```python
from build123d import *

# Parameters (mm, degrees)
SKETCH_1_W          = 100
SKETCH_1_H          = 35
EXTRUDE_1_DEPTH     = 1.6
CUT_EXTRUDE_1_DEPTH = 53.998207517
FILLET_1_R          = 3
SKETCH_3_W          = 12
SKETCH_3_H          = 6
EXTRUDE_2_DEPTH     = 6
SKETCH_4_R          = 3
EXTRUDE_3_DEPTH     = 10
SKETCH_5_W          = 4.5
SKETCH_5_H          = 6
SKETCH_5_W_2        = 5.403478788
SKETCH_5_H_2        = 11.06674021
EXTRUDE_4_DEPTH     = 2
SKETCH_6_W          = 7.585652914
SKETCH_6_H          = 2.805652448
SKETCH_6_W_2        = 13.612610022
EXTRUDE_5_DEPTH     = 2
SKETCH_7_W          = 9
SKETCH_7_H          = 4.5
EXTRUDE_6_DEPTH     = 6
CHAMFER_1_SIZE      = 2
SKETCH_9_R          = 0.65
CUT_EXTRUDE_2_DEPTH = 1
SWEEP_1_PROFILE_R   = 1.5
SKETCH_27_R         = 1.993301653
CUT_EXTRUDE_3_DEPTH = 1


with BuildPart() as part:
    # 草图1 → 凸台-拉伸1 (new body)
    with BuildSketch(Plane(origin=(0, 0, 0), x_dir=(1, 0, 0), z_dir=(0, 1, 0))):
        Rectangle(SKETCH_1_W, SKETCH_1_H)
    extrude(amount=EXTRUDE_1_DEPTH)

    # 草图2 → 切除-拉伸1 (cut, through all)
    with BuildSketch(Plane(origin=(0, 1.6, 0), x_dir=(1, 0, 0), z_dir=(0, 1, 0))):
        with BuildLine():
            Line((-49, 11), (-49, 15))
            ThreePointArc((-49, 15), (-47.5, 16.5), (-46, 15))
            Line((-46, 15), (-46, 11))
            ThreePointArc((-46, 11), (-47.5, 9.5), (-49, 11))
        make_face()
        with BuildLine():
            Line((49, 11), (49, 15))
            ThreePointArc((49, 15), (47.5, 16.5), (46, 15))
            Line((46, 15), (46, 11))
            ThreePointArc((46, 11), (47.5, 9.5), (49, 11))
        make_face()
        with BuildLine():
            Line((-49, -11), (-49, -15))
            ThreePointArc((-49, -15), (-47.5, -16.5), (-46, -15))
            Line((-46, -15), (-46, -11))
            ThreePointArc((-46, -11), (-47.5, -9.5), (-49, -11))
        make_face()
        with BuildLine():
            Line((49, -11), (49, -15))
            ThreePointArc((49, -15), (47.5, -16.5), (46, -15))
            Line((46, -15), (46, -11))
            ThreePointArc((46, -11), (47.5, -9.5), (49, -11))
        make_face()
    extrude(amount=-CUT_EXTRUDE_1_DEPTH, mode=Mode.SUBTRACT)

    # 圆角1
    fillet_1_edges = [part.edges().sort_by_distance(p)[0] for p in [
        (50, 0.8, 17.5),
        (-50, 0.8, 17.5),
        (-50, 0.8, -17.5),
        (50, 0.8, -17.5),
    ]]
    fillet(fillet_1_edges, radius=FILLET_1_R)

    # 草图3 → 凸台-拉伸2 (add)
    with BuildSketch(Plane(origin=(0, 1.6, 0), x_dir=(1, 0, 0), z_dir=(0, 1, 0))):
        with Locations((8, -14.5)):
            Rectangle(SKETCH_3_W, SKETCH_3_H)
    extrude(amount=EXTRUDE_2_DEPTH)

    # 草图4 → 凸台-拉伸3 (add)
    with BuildSketch(Plane(origin=(0, 7.6, 0), x_dir=(1, 0, 0), z_dir=(0, 1, 0))):
        with Locations(Location((8, -14.5, 0), (0, 0, 270))):
            Circle(SKETCH_4_R)
    extrude(amount=EXTRUDE_3_DEPTH)

    # 草图5 → 凸台-拉伸4 (add)
    with BuildSketch(Plane(origin=(0, 1.6, 0), x_dir=(1, 0, 0), z_dir=(0, 1, 0))):
        with Locations((-32.75, -2.5)):
            Rectangle(SKETCH_5_W, SKETCH_5_H)
        with Locations((-23.75, -2.5)):
            Rectangle(SKETCH_5_W, SKETCH_5_H)
        with Locations((-32.75, -12.5)):
            Rectangle(SKETCH_5_W, SKETCH_5_H)
        with Locations((-23.75, -12.5)):
            Rectangle(SKETCH_5_W, SKETCH_5_H)
        with Locations((-8.78065303, -7.299892016)):
            Rectangle(SKETCH_5_W_2, SKETCH_5_H_2)
        with Locations((23.75, -12.5)):
            Rectangle(SKETCH_5_W, SKETCH_5_H)
        with Locations((32.75, -12.5)):
            Rectangle(SKETCH_5_W, SKETCH_5_H)
        with Locations((32.75, -2.5)):
            Rectangle(SKETCH_5_W, SKETCH_5_H)
        with Locations((23.75, -2.5)):
            Rectangle(SKETCH_5_W, SKETCH_5_H)
    extrude(amount=EXTRUDE_4_DEPTH)

    # 草图6 → 凸台-拉伸5 (add)
    with BuildSketch(Plane(origin=(0, 1.6, 0), x_dir=(1, 0, 0), z_dir=(0, 1, 0))):
        with Locations((13.196957808, 8.988479137)):
            Rectangle(SKETCH_6_W, SKETCH_6_H)
        with Locations((-15.379131934, 8.988479137)):
            Rectangle(SKETCH_6_W_2, SKETCH_6_H)
    extrude(amount=EXTRUDE_5_DEPTH)

    # 草图7 → 凸台-拉伸6 (add)
    with BuildSketch(Plane(origin=(0, 1.6, 0), x_dir=(1, 0, 0), z_dir=(0, 1, 0))):
        with Locations((-28.25, 15.25)):
            Rectangle(SKETCH_7_W, SKETCH_7_H)
        with Locations((28.25, 15.25)):
            Rectangle(SKETCH_7_W, SKETCH_7_H)
        with Locations((-8.02152296, -15.25)):
            Rectangle(SKETCH_7_W, SKETCH_7_H)
    extrude(amount=EXTRUDE_6_DEPTH)

    # 倒角1
    chamfer_1_edges = [part.edges().sort_by_distance(p)[0] for p in [
        (-28.25, 7.6, -13),
        (28.25, 7.6, -13),
        (-8.02152296, 7.6, 13),
    ]]
    chamfer(chamfer_1_edges, length=CHAMFER_1_SIZE)

    # 草图9 → 切除-拉伸2 (cut)
    with BuildSketch(Plane(origin=(0, 7.6, 0), x_dir=(1, 0, 0), z_dir=(0, 1, 0))):
        with Locations(Location((-30.77012682, 16.126476079, 0), (0, 0, 270))):
            Circle(SKETCH_9_R)
        with Locations(Location((-25.898686841, 16.126476079, 0), (0, 0, 270))):
            Circle(SKETCH_9_R)
        with Locations(Location((25.614567714, 16.126476079, 0), (0, 0, 270))):
            Circle(SKETCH_9_R)
        with Locations(Location((30.638295355, 16.126476079, 0), (0, 0, 270))):
            Circle(SKETCH_9_R)
        with Locations(Location((-10.92906004, -16.309333864, 0), (0, 0, 270))):
            Circle(SKETCH_9_R)
        with Locations(Location((-5.225111254, -16.309333864, 0), (0, 0, 270))):
            Circle(SKETCH_9_R)
    extrude(amount=-CUT_EXTRUDE_2_DEPTH, mode=Mode.SUBTRACT)

    # 草图27 → 切除-拉伸3 (cut)
    with BuildSketch(Plane(origin=(0, 17.6, 0), x_dir=(1, 0, 0), z_dir=(0, 1, 0))):
        with Locations(Location((8, -14.5, 0), (0, 0, 270))):
            Circle(SKETCH_27_R)
    extrude(amount=-CUT_EXTRUDE_3_DEPTH, mode=Mode.SUBTRACT)


with BuildPart() as body_2:
    # 扫描1: sweep along a path in 草图10
    with BuildLine(Plane.XY.offset(14.5)) as sweep_1_path:
        Line((7.943335964, 14.862681463), (11, 26.862681463))
    # 扫描1 profile (on start of the path) → 扫描1 (sweep)
    with BuildSketch(Plane(origin=(7.943335964, 14.862681463, 14.5), x_dir=(0.9690562615876172, -0.24683995194828523, 0), z_dir=(0.24683995194828523, 0.9690562615876172, 0))):
        Circle(SWEEP_1_PROFILE_R)
    sweep(path=sweep_1_path.line)

    # 圆顶1: read off the stored shape, not the designer's step
    # 圆顶1 outline → 圆顶1 (revolve)
    with BuildSketch(Plane(origin=(3.904168632, -0.994477654, 14.5), x_dir=(0.9690562615876172, -0.2468399519482851, 0), z_dir=(0, 0, 1))):
        with BuildLine():
            Line((0, 28.746689146), (1.5, 28.746689145))
            ThreePointArc((1.5, 28.746689145), (1.060660172, 29.807349317), (0, 30.246689146))
            Line((0, 30.246689146), (0, 28.746689146))
        make_face()
    revolve(axis=Axis((3.904168632, -0.994477654, 14.5), (0.2468399519482851, 0.9690562615876172, 0)))


with BuildPart() as part_1:
    add(part.part)

    # 相交1: read off the stored shape, not the designer's step
    # 相交1: union body 2
    add(body_2.part)


solid = part_1.part
```
Input: part model. Units: mm. Frame: model coordinates. A direction names the side the tool comes from. Round coordinates to 2 decimals unless told otherwise and drop trailing zeros. Loops run counter-clockwise (first coordinate to the right, second up) from the corner with the lowest first, then second, coordinate; pieces in that order, holes last. Notation, with made-up numbers: (-18.75, 19) -> (3.25, 19) arc R26 ccw to (3.25, 39) -> close; hole circle Ø10 at (-36.75, 26.5). An arc over 180 degrees is marked (long way). Use one line per item in the form item = value. Start each with the question number.
Item 1: Section query B-B on x = -29. Return the cut outline in (y, z).
Item 2: Set-up query: faces 1 (the face through (-15, 3.6, -9)), 2 (the face through (33, 3.6, 2)), 3 (the face through (21.5, 3, 3)). Return all of +Z, -Z, +X, -X, +Y, -Y with unobstructed straight access to the full face (end or side cutting, diameter ignored); none if empty.
Item 3: Material intervals for L1, parallel to X at y = 2.75, z = 13.5; L2, parallel to Z at x = -34, y = 1.75; L3, parallel to Y at x = -25.5, z = 13, sorted ascending. Write a range as from..to.
Item 4: Section query A-A on z = -8.5. Return the cut outline in (x, y).
Item 5: Contact query for flat-ended pins moving along their axis: pin 1 Ø1.6 at (x, y) = (-14, 3) entering from -Z; pin 2 Ø0.6 at (y, z) = (2.5, 2) entering from -X; pin 3 Ø12 at (x, y) = (0.5, 15.5) entering from -Z; pin 4 Ø1 at (x, y) = (2.5, 9.5) entering from +Z. Output: stop coordinate, or through.
Item 6: Mould query, pull axis X, two halves, no side actions, for faces 4 (the face through (-24, 3.6, 12)), 5 (the face through (49.1, 0.81, -16.64)), 6 (the face through (-11.482, 3, 7)). Classes: pulls with the +X half, pulls with the -X half, needs draft (parallel to the pull), parting line crosses it, or undercut.
Item 7: Section query C-C on x = -41. Return the cut outline in (y, z).
Ans:
q1.outline = (0, -17.5) -> (7.6, -17.5) -> (7.6, -15) -> (5.6, -13) -> (1.6, -13) -> (1.6, 17.5) -> (0, 17.5) -> close
q2.face_1 = -Z, +X, -X, +Y
q2.face_2 = +Z, +X, -X, +Y
q2.face_3 = +Z, -Z, +Y
q3.L1 = -35..-30.5, -26..-21.5, -12.52..-3.52, 2..14, 21.5..26, 30.5..35
q3.L2 = -0.5..5.5, 9.5..15.5
q3.L3 = 0..3.6
q4.outline = (-50, 0) -> (50, 0) -> (50, 1.6) -> (16.99, 1.6) -> (16.99, 3.6) -> (9.4, 3.6) -> (9.4, 1.6) -> (-8.57, 1.6) -> (-8.57, 3.6) -> (-22.19, 3.6) -> (-22.19, 1.6) -> (-50, 1.6) -> close
q5.pin_1 = -10.39
q5.pin_2 = -35
q5.pin_3 = 11.9
q5.pin_4 = through
q6.face_4 = needs draft
q6.face_5 = pulls with the +X half
q6.face_6 = undercut
q7.outline = (0, -17.5) -> (1.6, -17.5) -> (1.6, 17.5) -> (0, 17.5) -> close
